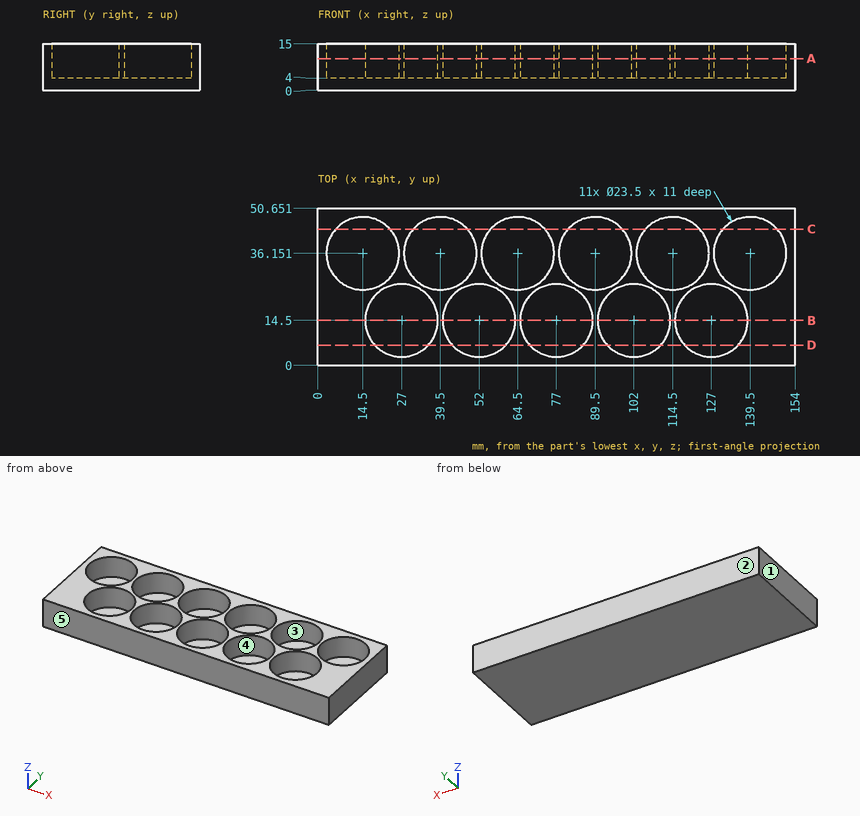
Source: three-view drawing plus pictorial views. Frame: mm from the lowest corner of the part. A direction names the side the tool comes from. Round coordinates to 2 decimals unless told otherwise and drop trailing zeros. Write each loop counter-clockwise with the first axis right and the second up, starting at its lowest first coordinate (ties: lowest second). Pieces come first, ordered by that corner, then holes. Notation, with made-up numbers: M 27,40 L 31,40 A21 ccw 31,57 Z; hole C 72,62.25 d4. An arc over 180 degrees is marked long. Use CSV: the item, a comma, the result in double quotes. Start each with the question number.
Q1. Pull-direction query (X, two-part tool) for the marked faces 1, 2 and 3; classes: +X half, -X half, draft (parallel to the pull), parting line (faces both ways), or undercut.
Q2. Cut plane B-B on y = 14.5. Output: boundary loops of the cut face in (x, z).
Q3. First-contact query: P1, Ø12, axis at x = 116, y = 34, coming from the +Z side. Flat tip, straight axial feed; report the tip coordinate or a pass-through.
Q4. Cut plane A-A on z = 10.25. Count the separate pieces of the cut face and the enclosed holes in it, plus the area to 3 significant figures.
Q5. Cut plane C-C on y = 44. Output: boundary loops of the cut face in (x, z).
Q6. Line query: line 1 (Y direction, x = 27, z = 9.5); line 2 (Y direction, x = 124.5, z = 14); line 3 (X direction, y = 20.5, z = 12.25). Output: solid intervals per line, ascending. Write a range as from..to.
Q7. Cut plane D-D on y = 6.5. Output: boundary loops of the cut face in (x, z).
Q8. Access query for the marked faces 4 and 5. Directions: +Z, -Z, +X, -X, +Y, -Y. A direction counts if a zero-diameter tool reaches every point of the face in a straight line with its end or side. Return the directions, or none.
Results found:
1,face 1,"-X half"
1,face 2,"draft"
1,face 3,"undercut"
2,outline,"M 0,0 L 154,0 L 154,15 L 138.75,15 L 138.75,4 L 115.25,4 L 115.25,15 L 113.75,15 L 113.75,4 L 90.25,4 L 90.25,15 L 88.75,15 L 88.75,4 L 65.25,4 L 65.25,15 L 63.75,15 L 63.75,4 L 40.25,4 L 40.25,15 L 38.75,15 L 38.75,4 L 15.25,4 L 15.25,15 L 0,15 Z"
3,P1,"z = 4"
4,separate pieces,"1"
4,enclosed holes,"11"
4,area,"3,030 mm^2"
5,outline,"M 0,0 L 154,0 L 154,15 L 148.24,15 L 148.24,4 L 130.76,4 L 130.76,15 L 123.24,15 L 123.24,4 L 105.76,4 L 105.76,15 L 98.24,15 L 98.24,4 L 80.76,4 L 80.76,15 L 73.24,15 L 73.24,4 L 55.76,4 L 55.76,15 L 48.24,15 L 48.24,4 L 30.76,4 L 30.76,15 L 23.24,15 L 23.24,4 L 5.76,4 L 5.76,15 L 0,15 Z"
6,line 1,"0..2.75, 26.25..50.65"
6,line 2,"0..3.02, 25.98..29.98, 42.32..50.65"
6,line 3,"0..16.9, 37.1..41.9, 62.1..66.9, 87.1..91.9, 112.1..116.9, 137.1..154"
7,outline,"M 0,0 L 154,0 L 154,15 L 135.61,15 L 135.61,4 L 118.39,4 L 118.39,15 L 110.61,15 L 110.61,4 L 93.39,4 L 93.39,15 L 85.61,15 L 85.61,4 L 68.39,4 L 68.39,15 L 60.61,15 L 60.61,4 L 43.39,4 L 43.39,15 L 35.61,15 L 35.61,4 L 18.39,4 L 18.39,15 L 0,15 Z"
8,face 4,"+Z"
8,face 5,"+Z, -Z, +X, -X, -Y"
